Geometry check sheet. Reference: the model listing, model coordinates, mm. Face numbers are marked on the shaded views. A direction names the side the tool comes from. Give positions to 0.01 mm unless a question says otherwise; leave off trailing zeros. Loops run counter-clockwise (first coordinate to the right, second up) from the corner with the lowest first, then second, coordinate; pieces in that order, holes last. Notation, with made-up numbers: (41.5, -1) -> (88.5, -1) arc R7 ccw to (88.5, 7) -> close; hole circle Ø8 at (51.5, -20.5). An arc over 180 degrees is marked (long way). Answer as a JSON object with one key per item and string values.
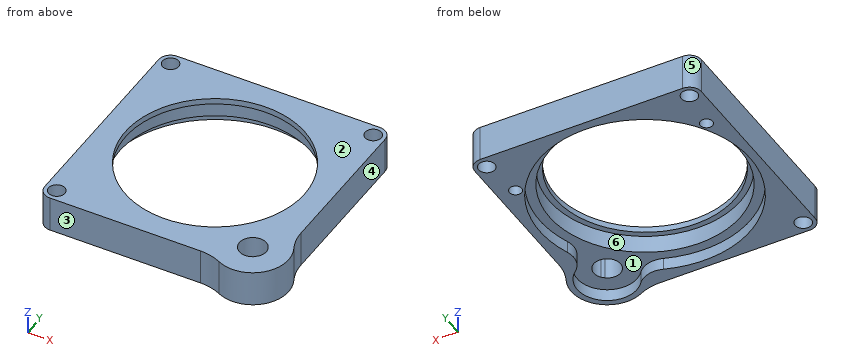
from build123d import *

# Parameters (mm, degrees)
SKETCH1_R                = 2.159
SKETCH1_R_2              = 28.5115
BOSS_EXTRUDE1_DEPTH      = 9.525
SKETCH1_4_R              = 28.5115
SKETCH1_4_R_2            = 23.8125
FLUSH_BEZEL_DEPTH        = 9.525
SKETCH1_5_R              = 28.5115
SKETCH1_5_R_2            = 23.8125
BOSS_EXTRUDE4_DEPTH      = 6.35
SKETCH2_R                = 25.3365
CUT_EXTRUDE1_DEPTH       = 7.35
CUT_EXTRUDE1_DEPTH_BACK  = 9.525
SKETCH3_R                = 28.5115
CUT_EXTRUDE2_DEPTH       = 7.35
SKETCH4_R                = 25.3365
SKETCH4_R_2              = 23.8125
BOSS_EXTRUDE7_DEPTH      = 1.5875
M6_CLEARANCE_HOLE1_D     = 7.14248
M6_CLEARANCE_HOLE1_DEPTH = 9.525
SKETCH8_R                = 2.159
BOSS_EXTRUDE8_DEPTH      = 9.525
SKETCH9_R                = 2.159
CUT_EXTRUDE3_DEPTH       = 10.525
SKETCH10_R               = 27.94
CUT_EXTRUDE4_DEPTH       = 3.2004
BOSS_EXTRUDE10_DEPTH     = 9.525
SKETCH12_R               = 7.9375
CUT_EXTRUDE5_DEPTH       = 3.2004
FILLET6_R                = 12.7
FILLET7_R                = 6.35
HOLE1_AT_2_COUNT         = 2
HOLE1_AT_2_PITCH         = 50.811879198
SKETCH18_W               = 1.5
SKETCH18_H               = 3.81
HOLE2_AT_2_COUNT         = 2
HOLE2_AT_2_PITCH         = 50.811879198


with BuildPart() as part:
    # Sketch1 → Boss-Extrude1 (new body)
    with BuildSketch(Plane.XY):
        with BuildLine():
            ThreePointArc((26.9875, -30.1625), (29.23256403, -29.23256403), (30.1625, -26.9875))
            Line((30.1625, -26.9875), (30.1625, 26.9875))
            ThreePointArc((30.1625, 26.9875), (29.23256403, 29.23256403), (26.9875, 30.1625))
            Line((26.9875, 30.1625), (-26.9875, 30.1625))
            ThreePointArc((-26.9875, 30.1625), (-29.23256403, 29.23256403), (-30.1625, 26.9875))
            Line((-30.1625, 26.9875), (-30.1625, -26.9875))
            ThreePointArc((-30.1625, -26.9875), (-29.23256403, -29.23256403), (-26.9875, -30.1625))
            Line((-26.9875, -30.1625), (26.9875, -30.1625))
        make_face()
        with Locations((26.9748, -26.9748)):
            Circle(SKETCH1_R, mode=Mode.SUBTRACT)
        with Locations((-26.9748, 26.9748)):
            Circle(SKETCH1_R, mode=Mode.SUBTRACT)
        Circle(SKETCH1_R_2, mode=Mode.SUBTRACT)
        with Locations((26.9748, 26.9748)):
            Circle(SKETCH1_R, mode=Mode.SUBTRACT)
    extrude(amount=BOSS_EXTRUDE1_DEPTH)

    # Sketch1_4 → Flush Bezel (add)
    with BuildSketch(Plane.XY):
        Circle(SKETCH1_4_R)
        Circle(SKETCH1_4_R_2, mode=Mode.SUBTRACT)
    extrude(amount=FLUSH_BEZEL_DEPTH)

    # Sketch1_5 → Boss-Extrude4 (add)
    with BuildSketch(Plane.XY):
        Circle(SKETCH1_5_R)
        Circle(SKETCH1_5_R_2, mode=Mode.SUBTRACT)
    extrude(amount=-BOSS_EXTRUDE4_DEPTH)

    # Sketch2 → Cut-Extrude1 (cut, two sides)
    with BuildSketch(Plane(origin=(0, 0, 0), x_dir=(-1, 0, 0), z_dir=(0, 0, -1))) as cut_extrude1_sk:
        Circle(SKETCH2_R)
    extrude(amount=CUT_EXTRUDE1_DEPTH, mode=Mode.SUBTRACT)
    extrude(cut_extrude1_sk.sketch, amount=-CUT_EXTRUDE1_DEPTH_BACK, mode=Mode.SUBTRACT)

    # Sketch3 → Cut-Extrude2 (cut, through all)
    with BuildSketch(Plane(origin=(0, 0, 0), x_dir=(-1, 0, 0), z_dir=(0, 0, -1))):
        Circle(SKETCH3_R)
    extrude(amount=CUT_EXTRUDE2_DEPTH, mode=Mode.SUBTRACT)

    # Sketch4 → Boss-Extrude7 (add)
    with BuildSketch(Plane.XY.offset(9.525)):
        Circle(SKETCH4_R)
        Circle(SKETCH4_R_2, mode=Mode.SUBTRACT)
    extrude(amount=-BOSS_EXTRUDE7_DEPTH)

    # M6 Clearance Hole1
    with Locations(Plane.XY.offset(9.525)):
        with Locations((22.98945567, -22.98945567)):
            Hole(M6_CLEARANCE_HOLE1_D / 2, depth=M6_CLEARANCE_HOLE1_DEPTH)

    # Sketch8 → Boss-Extrude8 (add, through all)
    with BuildSketch(Plane.XY.offset(9.525)):
        with Locations((26.9748, -26.9748)):
            Circle(SKETCH8_R)
    extrude(amount=-BOSS_EXTRUDE8_DEPTH)

    # Sketch9 → Cut-Extrude3 (cut, through all)
    with BuildSketch(Plane.XY.offset(9.525)):
        with Locations((-26.9748, -26.9748)):
            Circle(SKETCH9_R)
    extrude(amount=-CUT_EXTRUDE3_DEPTH, mode=Mode.SUBTRACT)

    # Sketch10 → Cut-Extrude4 (cut)
    with BuildSketch(Plane(origin=(0, 0, 0), x_dir=(-1, 0, 0), z_dir=(0, 0, -1))):
        Circle(SKETCH10_R)
    extrude(amount=-CUT_EXTRUDE4_DEPTH, mode=Mode.SUBTRACT)

    # Sketch13 → Boss-Extrude10 (add)
    with BuildSketch(Plane(origin=(0, 0, 0), x_dir=(-1, 0, 0), z_dir=(0, 0, -1))):
        with BuildLine():
            Line((-16.722633506, -30.1625), (-26.9875, -30.1625))
            ThreePointArc((-26.9875, -30.1625), (-29.23256403, -29.23256403), (-30.1625, -26.9875))
            Line((-30.1625, -26.9875), (-30.1625, -16.722633506))
            ThreePointArc((-30.1625, -16.722633506), (-29.724647761, -29.724647761), (-16.722633506, -30.1625))
        make_face()
    extrude(amount=-BOSS_EXTRUDE10_DEPTH)

    # Sketch12 → Cut-Extrude5 (cut)
    with BuildSketch(Plane(origin=(0, 0, 0), x_dir=(-1, 0, 0), z_dir=(0, 0, -1))):
        with Locations((-22.98945567, -22.98945567)):
            Circle(SKETCH12_R)
    extrude(amount=-CUT_EXTRUDE5_DEPTH, mode=Mode.SUBTRACT)

    # Fillet6
    fillet6_edges = [part.edges().sort_by_distance(p)[0] for p in [
        (30.1625, -16.722633506, 4.7625),
        (16.722633506, -30.1625, 4.7625),
    ]]
    fillet(fillet6_edges, radius=FILLET6_R)

    # Fillet7
    fillet7_edges = [part.edges().sort_by_distance(p)[0] for p in [
        (23.527276854, -15.070197206, 1.6002),
        (15.070197206, -23.527276854, 1.6002),
    ]]
    fillet(fillet7_edges, radius=FILLET7_R)

    # Sketch14 → Hole1 (revolve, cut)
    with BuildSketch(Plane(origin=(-25.405939599, 16.116198413, 0), x_dir=(0, 1, 0), z_dir=(1, 0, 0))):
        Polygon((0, 0), (0, 2.921), (1.4986, 2.921), (1.6383, 0), align=None)
    hole1 = revolve(axis=Axis((-25.405939599, 16.116198413, 110), (0, 0, -1)), mode=Mode.SUBTRACT)

    # Hole1 at 2: Hole1 ×2
    with Locations(*[(i * HOLE1_AT_2_PITCH, 0, 0) for i in range(1, HOLE1_AT_2_COUNT)]):
        add(hole1, mode=Mode.SUBTRACT)

    # Sketch18 → Hole2 (revolve, cut)
    with BuildSketch(Plane(origin=(25.405939599, 16.116198413, 2.921), x_dir=(0, 1, 0), z_dir=(1, 0, 0))):
        with Locations((0.75, 1.905)):
            Rectangle(SKETCH18_W, SKETCH18_H)
    hole2 = revolve(axis=Axis((25.405939599, 16.116198413, 112.921), (0, 0, -1)), mode=Mode.SUBTRACT)

    # Hole2 at 2: Hole2 ×2
    with Locations(*[(-i * HOLE2_AT_2_PITCH, 0, 0) for i in range(1, HOLE2_AT_2_COUNT)]):
        add(hole2, mode=Mode.SUBTRACT)


solid = part.part
1) Draft check along X on the marked faces 4, 5 and 6. Enter one of: pulls with the +X half, pulls with the -X half, needs draft (parallel to the pull), parting line crosses it, or undercut.
Geometry check:
{"face 4": "pulls with the +X half", "face 5": "pulls with the -X half", "face 6": "undercut"}
2) Material ranges on line 1 along Y through (x, z) = (-26, 6); line 2 along Y through (x, z) = (23, 7); line 3 along X through (y, z) = (0, 4.3), recorded low to high. Write a range as from..to.
Geometry check:
{"line 1": "y = -30.16..-28.9, -25.05..14.74, 17.49..25.05, 28.9..30.16", "line 2": "y = -32.51..-26.56, -19.42..-10.63, 10.63..30.16", "line 3": "x = -30.16..-25.34, 25.34..30.16"}
3) Depth check by flat-ended pin: P1, Ø5, axis at x = -26.97, y = -26.97, coming from the +Z side (3 decimals); P2, Ø2.5, axis at x = 25.41, y = 16.12, coming from the -Z side; P3, Ø12, axis at x = -18.5, y = 9, coming from the -Z side; P4, Ø2, axis at y = -16, z = 7, coming from the +X side. Enter the tip coordinate at first touch or a pass-through.
Geometry check:
{"P1": "stops at z = 9.525", "P2": "stops at z = 6.73", "P3": "stops at z = 3.2", "P4": "stops at x = 30.8"}
4) Section check C-C on z = 4.5. Count the separate pieces of the cut face and the enclosed holes in it, plus the area to 3 significant figures.
Geometry check:
{"separate pieces": "1", "enclosed holes": "7", "area": "1,560 mm2"}
5) Tool access check on the marked faces 1, 2 and 3. Record the directions out of +Z, -Z, +X, -X, +Y, -Y that give a thin tool (end or side, any length) a straight path to the whole face; none if there is none.
Geometry check:
{"face 1": "-Z", "face 2": "+Z, +X, -X, +Y, -Y", "face 3": "+Z, -Z, -X, -Y"}
6) Section check A-A on y = 0. Record the cut outline in (x, z) (1 decimal).
Geometry check:
{"outline": "(-30.2, 0) -> (-27.9, 0) -> (-27.9, 3.2) -> (-25.3, 3.2) -> (-25.3, 7.9) -> (-23.8, 7.9) -> (-23.8, 9.5) -> (-30.2, 9.5) -> close; (23.8, 7.9) -> (25.3, 7.9) -> (25.3, 3.2) -> (27.9, 3.2) -> (27.9, 0) -> (30.2, 0) -> (30.2, 9.5) -> (23.8, 9.5) -> close"}
